Build history of the part. All positions in model axes, mm. Face numbers are marked on the shaded views. A direction names the side the tool comes from. Round coordinates to 2 decimals unless told otherwise and drop trailing zeros. Write each loop counter-clockwise with the first axis right and the second up, starting at its lowest first coordinate (ties: lowest second). Pieces come first, ordered by that corner, then holes. Notation, with made-up numbers: M -30,64.25 L 5,64.25 A29 cw 5,93.25 Z; hole C -6.5,-0.75 d3. An arc over 180 degrees is marked long. Use a Markdown table: item, result.
from build123d import *

# Parameters (mm, degrees)
BOSS_EXTRU_1_DEPTH      = 675
ESQUISSE3_R             = 10.125
ESQUISSE3_R_2           = 12.5
ENL_V_MAT_EXTRU_1_DEPTH = 681.900139521
ENL_V_MAT_EXTRU_2_DEPTH = 681.900139521


with BuildPart() as part:
    # Esquisse2 → Boss.-Extru.1 (new body)
    with BuildSketch(Plane(origin=(0, 0, 0), x_dir=(1, 0, 0), z_dir=(0, 1, 0))):
        with BuildLine():
            Line((2, 0), (38, 0))
            ThreePointArc((38, 0), (39.414213562, 0.585786438), (40, 2))
            Line((40, 2), (40, 78))
            ThreePointArc((40, 78), (39.414213562, 79.414213562), (38, 80))
            Line((38, 80), (2, 80))
            ThreePointArc((2, 80), (0.585786438, 79.414213562), (0, 78))
            Line((0, 78), (0, 2))
            ThreePointArc((0, 2), (0.585786438, 0.585786438), (2, 0))
        make_face()
        with BuildLine():
            Line((6, 4), (34, 4))
            ThreePointArc((34, 4), (35.414213562, 4.585786438), (36, 6))
            Line((36, 6), (36, 74))
            ThreePointArc((36, 74), (35.414213562, 75.414213562), (34, 76))
            Line((34, 76), (6, 76))
            ThreePointArc((6, 76), (4.585786438, 75.414213562), (4, 74))
            Line((4, 74), (4, 6))
            ThreePointArc((4, 6), (4.585786438, 4.585786438), (6, 4))
        make_face(mode=Mode.SUBTRACT)
    extrude(amount=BOSS_EXTRU_1_DEPTH)

    # Esquisse3 → Enlèv. mat.-Extru.1 (cut, through all)
    with BuildSketch(Plane(origin=(40, 0, 0), x_dir=(0, 0, -1), z_dir=(1, 0, 0))):
        with Locations((40, 60)):
            Circle(ESQUISSE3_R)
        with Locations((40, 635)):
            Circle(ESQUISSE3_R_2)
    extrude(amount=-ENL_V_MAT_EXTRU_1_DEPTH, mode=Mode.SUBTRACT)

    # Esquisse4 → Enlèv. mat.-Extru.2 (cut, through all)
    with BuildSketch(Plane.XY):
        Polygon((0, 675), (40, 675), (40, 535), (0, 465.717967697), align=None)
    extrude(amount=-ENL_V_MAT_EXTRU_2_DEPTH, mode=Mode.SUBTRACT)


solid = part.part
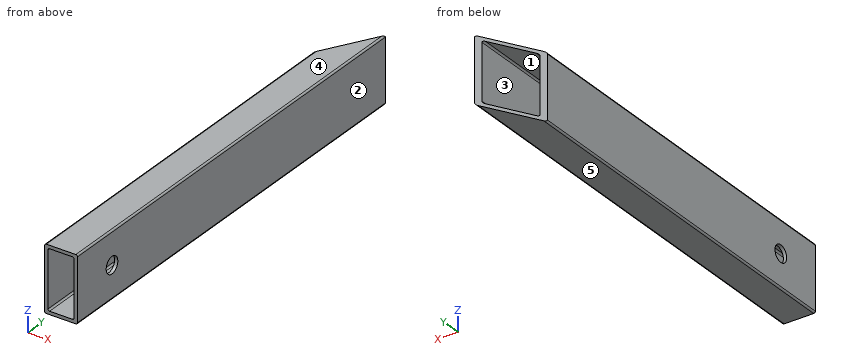
Q1. Which spindle directions (+Z, -Z, +X, -X, +Y, -Y) get a long thin tool onto all of the face, cutting with end or side? Do the marked faces 1 and 2. Say none if no direction does.
Response values:
| item | result |
|---|---|
| face 1 | +Y, -Y |
| face 2 | +Z, -Z, +X, +Y, -Y |
Q2. Cut at B-B on z = -68. Give the cut face in (x, y).
Response values:
| item | result |
|---|---|
| outline | M 0,0 L 4,0 L 4,472.65 L 0,465.72 Z; M 36,0 L 40,0 L 40,535 L 36,528.07 Z |
Q3. Two-plate mould, pull along Z, no slides. Class the marked faces 3, 4 and 5: +Z half, -Z half, draft (parallel to the pull), parting line (faces both ways), or undercut.
Response values:
| item | result |
|---|---|
| face 3 | undercut |
| face 4 | +Z half |
| face 5 | -Z half |
Q4. Cut at D-D on x = 22.5. Give the cut face in (y, z).
Response values:
| item | result |
|---|---|
| outline | M 0,-80 L 504.69,-80 L 504.69,-76 L 0,-76 Z; M 0,-4 L 504.69,-4 L 504.69,0 L 0,0 Z |
Q5. Cut at A-A on y = 398.5. Give the cut face in (x, z), and give its area (3 significant figures).
Response values:
| item | result |
|---|---|
| outline | M 0,-78 A2 ccw 2,-80 L 38,-80 A2 ccw 40,-78 L 40,-2 A2 ccw 38,0 L 2,0 A2 ccw 0,-2 Z; hole M 4,-74 A2 ccw 6,-76 L 34,-76 A2 ccw 36,-74 L 36,-6 A2 ccw 34,-4 L 6,-4 A2 ccw 4,-6 Z |
| area | 896 mm2 |
Q6. Drill centre lines: L1, parallel to Z at x = 17, y = 454.5; L2, parallel to X at y = 447.5, z = -9; L3, parallel to Y at x = 2, z = -40 (3 decimals). Where is each one in solid material? Low to high.
Response values:
| item | result |
|---|---|
| L1 | z = -80 to -76, -4 to 0 |
| L2 | x = 0 to 4, 36 to 40 |
| L3 | y = 0 to 49.875, 70.125 to 469.182 |
Q7. Cut at C-C on y = 60. Give the cut face in (x, z) (3 decimals).
Response values:
| item | result |
|---|---|
| outline | M 0,-78 A2 ccw 2,-80 L 38,-80 A2 ccw 40,-78 L 40,-50.125 L 36,-50.125 L 36,-74 A2 cw 34,-76 L 6,-76 A2 cw 4,-74 L 4,-50.125 L 0,-50.125 Z; M 0,-29.875 L 4,-29.875 L 4,-6 A2 cw 6,-4 L 34,-4 A2 cw 36,-6 L 36,-29.875 L 40,-29.875 L 40,-2 A2 ccw 38,0 L 2,0 A2 ccw 0,-2 Z |
